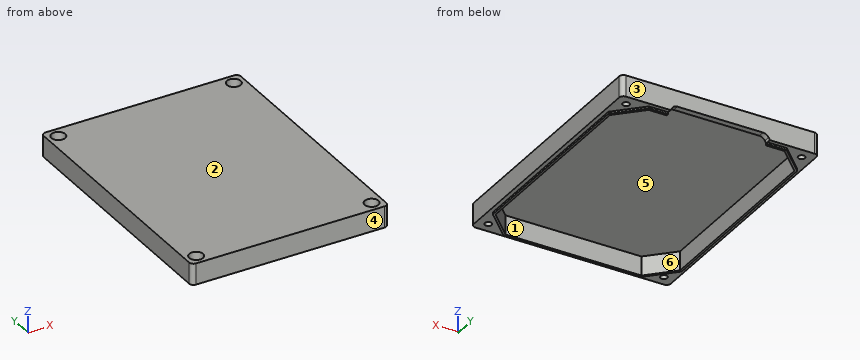
```python
from build123d import *

# Parameters (mm, degrees)
ESQUISSE1_R       = 1.6
WALLS_DEPTH       = 10
CENTRAGE_DEPTH    = 1
PASSAGE_CMC_REACH = 130.98
COUVERCLE_DEPTH   = 2
PASSAGE_M3_START  = -5
ESQUISSE5_R       = 3.25
ESQUISSE5_R_2     = 1.6
PASSAGE_M3_DEPTH  = 5


with BuildPart() as part:
    # Esquisse1 → Walls (new body)
    with BuildSketch(Plane.XY):
        with BuildLine():
            Line((-44.32, 60.43), (44.32, 60.43))
            ThreePointArc((44.32, 60.43), (45.734213562, 59.844213562), (46.32, 58.43))
            Line((46.32, 58.43), (46.32, -57.53))
            ThreePointArc((46.32, -57.53), (45.734213562, -58.944213562), (44.32, -59.53))
            Line((44.32, -59.53), (-44.32, -59.53))
            ThreePointArc((-44.32, -59.53), (-45.734213562, -58.944213562), (-46.32, -57.53))
            Line((-46.32, -57.53), (-46.32, 58.43))
            ThreePointArc((-46.32, 58.43), (-45.734213562, 59.844213562), (-44.32, 60.43))
        make_face()
        with Locations((-41.248784258, -54.458784258)):
            Circle(ESQUISSE1_R, mode=Mode.SUBTRACT)
        with Locations((41.248784258, -54.458784258)):
            Circle(ESQUISSE1_R, mode=Mode.SUBTRACT)
        with Locations((41.248784258, 55.358784258)):
            Circle(ESQUISSE1_R, mode=Mode.SUBTRACT)
        with Locations((-41.248784258, 55.358784258)):
            Circle(ESQUISSE1_R, mode=Mode.SUBTRACT)
        Polygon((-43.37, 46.065786438), (-31.955786438, 57.48), (31.955786438, 57.48), (43.37, 46.065786438), (43.37, -45.165786438), (31.955786438, -56.58), (-31.955786438, -56.58), (-43.37, -45.165786438), align=None, mode=Mode.SUBTRACT)
    extrude(amount=WALLS_DEPTH)

    # Esquisse1<5> → Centrage (add)
    with BuildSketch(Plane.XY):
        Polygon((-44.37, 46.48), (-32.37, 58.48), (32.37, 58.48), (44.37, 46.48), (44.37, -45.58), (32.37, -57.58), (-32.37, -57.58), (-44.37, -45.58), align=None)
        Polygon((-31.955786438, -56.58), (-43.37, -45.165786438), (-43.37, 46.065786438), (-31.955786438, 57.48), (31.955786438, 57.48), (43.37, 46.065786438), (43.37, -45.165786438), (31.955786438, -56.58), align=None, mode=Mode.SUBTRACT)
    extrude(amount=-CENTRAGE_DEPTH)

    # Esquisse2 → Passage_CMC (cut, up to next)
    with BuildSketch(Plane(origin=(0, 60.43, 0), x_dir=(1, 0, 0), z_dir=(0, 1, 0)), mode=Mode.PRIVATE) as passage_cmc_sk1:
        with BuildLine():
            Line((-23.35, 1), (23.35, 1))
            Line((23.35, 1), (23.35, 0))
            Line((23.35, 0), (22.72, -1.1))
            ThreePointArc((22.72, -1.1), (21.621090793, -2.198557375), (20.12, -2.6))
            Line((20.12, -2.6), (-20.12, -2.6))
            ThreePointArc((-20.12, -2.6), (-21.621090793, -2.198557375), (-22.72, -1.1))
            Line((-22.72, -1.1), (-23.35, 0))
            Line((-23.35, 0), (-23.35, 1))
        make_face()
    passage_cmc_tool1 = extrude(passage_cmc_sk1.sketch, amount=-PASSAGE_CMC_REACH, mode=Mode.PRIVATE) & part.part
    add(passage_cmc_tool1.solids().sort_by_distance((0, 60.43, 0.768983))[0], mode=Mode.SUBTRACT)

    # Esquisse4 → Couvercle (add)
    with BuildSketch(Plane.XY.offset(10)):
        Polygon((-43.37, -45.165786438), (-43.37, 46.065786438), (-31.955786438, 57.48), (31.955786438, 57.48), (43.37, 46.065786438), (43.37, -45.165786438), (31.955786438, -56.58), (-31.955786438, -56.58), align=None)
    extrude(amount=-COUVERCLE_DEPTH)

    # Esquisse5 → Passage_M3 (cut)
    # profile 1 of 4: a face of its own
    with BuildSketch(Plane.XY.offset(10).offset(PASSAGE_M3_START)):
        with Locations((-41.248784258, -54.458784258)):
            Circle(ESQUISSE5_R)
        with Locations((-41.248784258, -54.458784258)):
            Circle(ESQUISSE5_R_2, mode=Mode.SUBTRACT)
    # profile 2 of 4: a face of its own
    with BuildSketch(Plane.XY.offset(10).offset(PASSAGE_M3_START)):
        with Locations((-41.248784258, 55.358784258)):
            Circle(ESQUISSE5_R)
        with Locations((-41.248784258, 55.358784258)):
            Circle(ESQUISSE5_R_2, mode=Mode.SUBTRACT)
    # profile 3 of 4: a face of its own
    with BuildSketch(Plane.XY.offset(10).offset(PASSAGE_M3_START)):
        with Locations(Location((41.248784258, 55.358784258, 0), (0, 0, 180))):
            Circle(ESQUISSE5_R)
        with Locations(Location((41.248784258, 55.358784258, 0), (0, 0, 180))):
            Circle(ESQUISSE5_R_2, mode=Mode.SUBTRACT)
    # profile 4 of 4: a face of its own
    with BuildSketch(Plane.XY.offset(10).offset(PASSAGE_M3_START)):
        with Locations(Location((41.248784258, -54.458784258, 0), (0, 0, 180))):
            Circle(ESQUISSE5_R)
        with Locations(Location((41.248784258, -54.458784258, 0), (0, 0, 180))):
            Circle(ESQUISSE5_R_2, mode=Mode.SUBTRACT)
    extrude(amount=PASSAGE_M3_DEPTH, mode=Mode.SUBTRACT)


solid = part.part
```
Here's how the part is built. I have some questions about the finished solid (model axes, mm). Face numbers are marked on the shaded views. A direction names the side the tool comes from. Coordinates: 2 decimals unless noted, no trailing zeros. Order: outer loops, then holes, each group sorted by start corner. A loop starts at its lowest first (then second) coordinate and runs counter-clockwise, first axis right, second up. Notation, with made-up numbers: (34, 81.25) -> (48, 81.25) arc R15 cw to (48, 95.25) -> close; hole circle Ø9 at (39, 18.5). An arc over 180 degrees is marked (long way). Return JSON: item names as keys, results as strings.
1) Thinking about a two-plate mould opening in Y: for the marked faces 3, 4, 5 and 6, which applies, +Y half, -Y half, draft (parallel to the pull), parting line (faces both ways), or undercut?
Conclusion:
{"face 3": "+Y half", "face 4": "-Y half", "face 5": "undercut", "face 6": "undercut"}
2) I'm going to push flat-ended pins straight in: P1, Ø2.5, axis at x = 4, y = 59.5, coming from the -Z side; P2, Ø5, axis at x = 41.5, y = -54, coming from the +Z side; P3, Ø0.5, axis at y = -0.5, z = -0.5, coming from the -X side; P4, Ø3, axis at x = -41.25, y = 55.36, coming from the +Z side. Where does each tip first touch, or does it pass through?
Conclusion:
{"P1": "stops at z = 2.6", "P2": "stops at z = 5", "P3": "stops at x = -44.37", "P4": "passes through"}
3) If we section it at B-B on z = 6.25: List the corners of the cut face in (x, y) for me, plus the area to 3 significant figures.
Conclusion:
{"outline": "(-46.32, -57.53) arc R2 ccw to (-44.32, -59.53) -> (44.32, -59.53) arc R2 ccw to (46.32, -57.53) -> (46.32, 58.43) arc R2 ccw to (44.32, 60.43) -> (-44.32, 60.43) arc R2 ccw to (-46.32, 58.43) -> close; hole circle Ø6.5 at (-41.25, -54.46); hole circle Ø6.5 at (-41.25, 55.36); hole (-43.37, -45.17) -> (-31.96, -56.58) -> (31.96, -56.58) -> (43.37, -45.17) -> (43.37, 46.07) -> (31.96, 57.48) -> (-31.96, 57.48) -> (-43.37, 46.07) -> close; hole circle Ø6.5 at (41.25, -54.46); hole circle Ø6.5 at (41.25, 55.36)", "area": "1,340 mm²"}
4) On a 3-axis mill with a long thin cutter (end or side, diameter ignored), from which of +Z, -Z, +X, -X, +Y, -Y can I reach the whole of each face in a straight line? I mean the marked faces 1 and 2. Say none if no direction works.
Conclusion:
{"face 1": "-Z", "face 2": "+Z, +X, -X, +Y, -Y"}
5) If I drill on probe 1 along Y at (x, z) = (-23.5, 0.25); probe 2 along X at (y, z) = (-7, 6.25); probe 3 along Y at (x, z) = (-42, 4), over which ranges is the centre line in solid material (lowest first)?
Conclusion:
{"probe 1": "y = -59.53 to -56.58, 57.48 to 60.43", "probe 2": "x = -46.32 to -43.37, 43.37 to 46.32", "probe 3": "y = -59.53 to -55.87, -53.05 to -46.54, 47.44 to 53.95, 56.77 to 60.43"}
6) If we section it at C-C on x = -16.5: List the corners of the cut face in (y, z) for me.
Conclusion:
{"outline": "(-59.53, 0) -> (-57.58, 0) -> (-57.58, -1) -> (-56.58, -1) -> (-56.58, 8) -> (57.48, 8) -> (57.48, 2.6) -> (60.43, 2.6) -> (60.43, 10) -> (-59.53, 10) -> close"}
7) If we section it at D-D on y = 48: List the corners of the cut face in (x, z) for me.
Conclusion:
{"outline": "(-46.32, 0) -> (-42.85, 0) -> (-42.85, -1) -> (-41.44, -1) -> (-41.44, 8) -> (41.44, 8) -> (41.44, -1) -> (42.85, -1) -> (42.85, 0) -> (46.32, 0) -> (46.32, 10) -> (-46.32, 10) -> close"}
8) If we section it at A-A on y = -5: List the corners of the cut face in (x, z) for me, plus the area to 3 significant figures.
Conclusion:
{"outline": "(-46.32, 0) -> (-44.37, 0) -> (-44.37, -1) -> (-43.37, -1) -> (-43.37, 8) -> (43.37, 8) -> (43.37, -1) -> (44.37, -1) -> (44.37, 0) -> (46.32, 0) -> (46.32, 10) -> (-46.32, 10) -> close", "area": "234 mm²"}
